Design review of the part built by this model. Coordinates are the model's own, in mm. Give positions to 0.01 mm unless a question says otherwise; leave off trailing zeros. Loops run counter-clockwise (first coordinate to the right, second up) from the corner with the lowest first, then second, coordinate; pieces in that order, holes last. Notation, with made-up numbers: M 89.5,-34 L 133.5,-34 A23 cw 133.5,-8 Z; hole C 80,6 d8. An arc over 180 degrees is marked long. Use a Markdown table: item, result. Add a question column.
(1) Add section D-D, the plane x = 50. Give the boundary of the cut face in (y, z).
(2) Add section C-C, the plane y = -8.25. Give the boundary of the cut face in (x, z).
(3) Add section B-B, the plane z = 21. Give the boundary of the cut face in (x, y), then the cut area to 3 significant figures.
(4) Add section A-A, the plane x = 29. Give the boundary of the cut face in (y, z), then the cut area to 3 significant figures.
(5) Insertion check: pin 1 Ø12 at (y, z) = (-3.5, 17) entering from +X; pin 2 Ø3 at (y, z) = (-10, 32) entering from +X; pin 3 Ø2 at (y, z) = (-20.5, 13) entering from +X. Each pin has a flat end and moves straight along its axis. Give the tip position at first contact, or say it passes through.
(6) For probe 1 along Z at (x, y) = (42.5, -9.25); probe 2 along Y at (x, z) = (22.5, 25); probe 3 along X at (y, z) = (-13.75, 13.5), list the stretches that pass through material, from the lowest coordinate up.
```python
from build123d import *

# Parameters (mm, degrees)
F1_DEPTH = 25.4
F2_DEPTH = 25.4
F6_DEPTH = 15.875


with BuildPart() as f1:
    # F0 (on Front) → F1 (new body)
    with BuildSketch(Plane.XZ):
        Polygon((15.875, 19.05), (0, 0), (63.5, 0), (47.625, 19.05), align=None)
    extrude(amount=F1_DEPTH)

    # F0 (on Front) → F2 (join)
    with BuildSketch(Plane.XZ):
        Polygon((15.875, 19.05), (0, 0), (63.5, 0), (47.625, 19.05), align=None)
        Polygon((31.75, 38.1), (15.875, 19.05), (47.625, 19.05), align=None)
    extrude(amount=F2_DEPTH)

    # F5 (on 3pt) → F6 (cut, symmetric)
    with BuildSketch(Plane.YZ.offset(31.75)):
        Polygon((-25.4, 19.05), (-12.7, 38.1), (-25.4, 38.1), align=None)
    extrude(amount=F6_DEPTH, both=True, mode=Mode.SUBTRACT)


solid = f1.part
```
Established:
| question | item | result |
|---|---|---|
| 1 | outline | M -25.4,0 L 0,0 L 0,16.2 L -25.4,16.2 Z |
| 2 | outline | M 0,0 L 63.5,0 L 31.75,38.1 Z |
| 3 | outline | M 17.5,-24.1 L 46,-24.1 L 46,0 L 17.5,0 Z |
| 3 | area | 687 mm^2 |
| 4 | outline | M -25.4,0 L 0,0 L 0,34.8 L -14.9,34.8 L -25.4,19.05 Z |
| 4 | area | 801 mm^2 |
| 5 | pin 1 | x = 54.33 |
| 5 | pin 2 | x = 38.08 |
| 5 | pin 3 | x = 53.5 |
| 6 | probe 1 | 0 to 25.2 |
| 6 | probe 2 | -21.43 to 0 |
| 6 | probe 3 | 11.25 to 52.25 |
